from build123d import *

# Parameters (mm, degrees)
F1_DEPTH    = 10
F2_T1_DEPTH = 20


# Not quite as in the source:
# - a fillet or chamfer that OpenCascade refuses, or shapes differently, is made with other operations: its cross-section is extruded or revolved along the edge and cut away or added


with BuildPart() as f1:
    # F0 (on Top) → F1 (new body)
    with BuildSketch(Plane.XY):
        with BuildLine():
            ThreePointArc((-2.2298651391, -0.300335581), (-0.1505048785, 2.2449606414), (2.25, 0))
            Line((2.25, 0), (2.25, -15))
            Line((2.25, -15), (6.25, -15))
            Line((6.25, -15), (6.25, 0))
            ThreePointArc((6.25, 0), (-0.418069107, 6.2360017817), (-6.194069831, -0.8342655028))
            Line((-6.194069831, -0.8342655028), (-4.2142046918, -15.5339299218))
            Line((-4.2142046918, -15.5339299218), (-0.25, -15))
            Line((-0.25, -15), (-2.2298651391, -0.300335581))
        make_face()
    extrude(amount=F1_DEPTH)

    # F2: fillet of radius 2 on 2 edges, made by hand

    # F2_s2 → F2_t1 (cut)
    with BuildSketch(Plane.XY.offset(-5)):
        with BuildLine():
            add(Edge.make_bspline(
                [(-2.2321023459, -15.2669649609), (-0.25, -15), (-0.5169649609, -13.0178976541)],
                knots=[0, 0, 0, 1, 1, 1], degree=2, weights=[1, 1, 1]))
            Line((-0.5169649609, -13.0178976541), (-0.25, -15))
            Line((-0.25, -15), (-2.2321023459, -15.2669649609))
        make_face()
        with BuildLine():
            add(Edge.make_bspline(
                [(2.25, -13), (2.25, -15), (4.25, -15)],
                knots=[0, 0, 0, 1, 1, 1], degree=2, weights=[1, 1, 1]))
            Line((4.25, -15), (2.25, -15))
            Line((2.25, -15), (2.25, -13))
        make_face()
    extrude(amount=F2_T1_DEPTH, mode=Mode.SUBTRACT)


solid = f1.part
Input: part model. Units: mm. Frame: model coordinates. A direction names the side the tool comes from. Give positions to 0.01 mm unless a question says otherwise; leave off trailing zeros. Loops run counter-clockwise (first coordinate to the right, second up) from the corner with the lowest first, then second, coordinate; pieces in that order, holes last. Notation, with made-up numbers: (64.25, 12.25) - (118.25, 12.25) arc R32 ccw to (118.25, 45.25) - close; hole circle Ø9 at (53, -30). An arc over 180 degrees is marked (long way). Use CSV: the item, a comma, the result in double quotes. Start each with the question number.
Item 1: Reachability of faces 5 (the flat face through (6.25, -8, 5)), 6 (the flat face through (2.25, -6, 5)), 7 (the flat face through (5, -15, 5)), 8 (the flat face through (-1.36, -6.75, 4.93)) from +Z, -Z, +X, -X, +Y, -Y: full face, straight path, thin tool, end or side. Return the list, or none.
Item 2: Line query: line 1 (X direction, y = -9, z = 1.25); line 2 (X direction, y = -10.5, z = 8.5); line 3 (Y direction, x = -3.5, z = 6.5). Output: solid intervals per line, ascending.
Item 3: Section C-C on x = -4.75. Return loops of the section in (y, z), then the cut area to 3 significant figures.
Item 4: Contact query for flat-ended pins moving along their axis: P1, Ø1, axis at x = 3.5, z = 5, coming from the +Y side; P2, Ø1.5, axis at x = 2.5, y = -4.5, coming from the -Z side; P3, Ø2, axis at y = 3.5, z = 6.5, coming from the -X side; P4, Ø0.6, axis at x = 5.5, z = 6, coming from the -Y side. Output: stop coordinate, or through.
Item 5: Section A-A on y = -3.5. Return loops of the section in (x, z).
Item 6: Section B-B on x = 0. Return loops of the section in (y, z), then the cut area to 3 significant figures.
Item 7: Mould query, pull axis X, two halves, no side actions, for faces 1 (the cylindrical face through (-0.2, 2.24, 4.93)), 2 (the flat face through (3, -4, 10)), 3 (the cylindrical face through (-0.275, 6.244, 4.93)), 4 (the flat face through (-5.22, -8.08, 4.93)). Classes: pulls with the +X half, pulls with the -X half, needs draft (parallel to the pull), parting line crosses it, or undercut.
Ans:
1,face 5,"+Z, -Z, +X, +Y, -Y"
1,face 6,"+Z, -Z, -Y"
1,face 7,"+Z, -Z, +X, -Y"
1,face 8,"+Z, -Z"
2,line 1,"x = -5.09 to -1.06, 2.25 to 6.25"
2,line 2,"x = -4.89 to -0.86, 2.25 to 6.25"
2,line 3,"y = -15.44 to 5.18"
3,outline,"(-11.56, 0) - (4.06, 0) - (4.06, 10) - (-11.56, 10) - close"
3,area,"156 mm2"
4,P1,"stops at y = 5.48"
4,P2,"stops at z = 0"
4,P3,"stops at x = -5.73"
4,P4,"stops at y = -15"
5,outline,"(-5.84, 0) - (-1.8, 0) - (-1.8, 10) - (-5.84, 10) - close; (2.25, 0) - (6.25, 0) - (6.25, 10) - (2.25, 10) - close"
6,outline,"(2.25, 0) - (6.25, 0) - (6.25, 10) - (2.25, 10) - close"
6,area,"40.0 mm2"
7,face 1,"undercut"
7,face 2,"needs draft"
7,face 3,"parting line crosses it"
7,face 4,"pulls with the -X half"
